Autodesk Inventor part; units mm, degrees
ref_plane "YZ Plane" through (0, 0, 0) normal (1, 0, 0) x (0, 1, 0)
ref_plane "XZ Plane" through (0, 0, 0) normal (0, 1, 0) x (-1, 0, 0)
ref_plane "XY Plane" through (0, 0, 0) normal (0, 0, 1) x (1, 0, 0)
sketch "Sketch1" plane through (0, 0, 0) normal (0, 1, 0) x (-1, 0, 0)
  line L0 (-63.881, 88.9) -> (63.881, 88.9)
  line L1 (63.881, 88.9) -> (63.881, -88.9)
  line L2 (63.881, -88.9) -> (-63.881, -88.9)
  line L3 (-63.881, -88.9) -> (-63.881, 88.9)
  line L4 (-63.881, 88.9) -> (63.881, -88.9) construction
  line L5 (63.881, 88.9) -> (-63.881, -88.9) construction
  point P0 (0, 0)
  dimension "d0" = 127.762
  dimension "d1" = 177.8
extrude "Extrusion1" add sketch "Sketch1" along normal blind 6.35
sketch "Sketch4" plane through (0, 0, 0) normal (0, -1, 0) x (1, 0, 0)
  line L0 (63.881, 88.9) -> (-63.881, 88.9)
  line L1 (-63.881, 88.9) -> (-63.881, -88.9)
  line L2 (63.881, 88.9) -> (-63.881, 88.9)
  line L3 (-63.881, 88.9) -> (-63.881, 76.2)
  line L4 (-63.881, 76.2) -> (63.881, 76.2)
  line L5 (63.881, 76.2) -> (63.881, 88.9)
  point P0 (0, 0)
  point P1 (-59.9113, 88.9)
  point P2 (-63.881, 84.7576)
  dimension "d9" = 12.7
extrude "Extrusion4" cut sketch "Sketch4" against normal blind 6.35
sketch "Sketch6" plane through (0, 0, 0) normal (0, -1, 0) x (1, 0, 0)
  circle A0 centre (-11.3792, 59.9948) radius 1.3716
  circle A1 centre (20.701, 61.722) radius 1.1303
  circle A2 centre (-11.303, 7.62) radius 1.1303
  circle A3 centre (60.071, 7.62) radius 1.1303
  circle A4 centre (-51.181, -41.91) radius 1.4986
  circle A5 centre (50.419, -41.91) radius 1.4986
  circle A6 centre (50.419, -68.58) radius 1.4986
  circle A7 centre (-51.181, -68.58) radius 1.4986
  point P0 (0, 0)
  point P1 (63.881, 76.2)
  dimension "d24" = 2.7432
  dimension "d26" = 2.2606
  dimension "d33" = 2.2606
  dimension "d34" = 2.2606
  dimension "d48" = 2.9972
  dimension "d49" = 2.9972
  dimension "d63" = 2.9972
  dimension "d64" = 2.9972
sketch "Sketch7" plane through (0, 6.35, 0) normal (0, 1, 0) x (1, 0, 0)
  line L0 (-63.881, -76.2) -> (63.881, -76.2)
  line L1 (-63.881, -76.2) -> (-63.881, 88.9)
  line L2 (63.881, -76.2) -> (-63.881, -76.2)
  line L3 (-63.881, -76.2) -> (-63.881, -69.85)
  line L4 (-63.881, -69.85) -> (63.881, -69.85)
  line L5 (63.881, -69.85) -> (63.881, -76.2)
  point P0 (0, 0)
  dimension "d204" = 6.35
extrude "Extrusion7" cut sketch "Sketch7" against normal blind 25.4
sketch "Sketch8" plane through (0, 0, 0) normal (0, -1, 0) x (1, 0, 0)
  circle A0 centre (-20.701, -67.31) radius 1.4986
  circle A1 centre (-20.701, -50.9524) radius 1.4986
  circle A2 centre (16.891, -50.9524) radius 1.4986
  circle A3 centre (16.891, -67.31) radius 1.4986
  point P0 (0, 0)
  point P1 (-63.881, -88.9)
  dimension "d213" = 2.9972
  dimension "d216" = 2.9972
  dimension "d217" = 2.9972
  dimension "d218" = 2.9972
extrude "Extrusion8" cut sketch "Sketch8" against normal blind 25.4
sketch "Sketch9" plane through (0, 6.35, 0) normal (0, 1, 0) x (1, 0, 0)
  point P0 (0, 0)
sketch "Sketch10" plane through (0, 6.35, 0) normal (0, 1, 0) x (1, 0, 0)
  circle A0 centre (-20.701, 67.31) radius 1.4986
  circle A1 centre (-20.701, 67.31) radius 6.35
  circle A2 centre (16.891, 67.31) radius 1.4986
  circle A3 centre (16.891, 67.31) radius 6.35
  circle A4 centre (16.891, 50.9524) radius 1.4986
  circle A5 centre (16.891, 50.9524) radius 6.35
  circle A6 centre (-20.701, 50.9524) radius 1.4986
  circle A7 centre (-20.701, 50.9524) radius 6.35
  point P0 (0, 0)
  dimension "d221" = 12.7
  dimension "d222" = 12.7
  dimension "d223" = 12.7
  dimension "d224" = 12.7
extrude "Extrusion9" cut sketch "Sketch10" against normal blind 3.175
extrude "Extrusion14" cut sketch "Sketch6" against normal blind 6.35 contours A4 | A5 | A6 | A7
sketch "Sketch13" plane through (0, 0, 0) normal (0, -1, 0) x (1, 0, 0)
  circle A0 centre (-51.181, -41.91) radius 1.4986
  circle A1 centre (-51.181, -41.91) radius 6.35
  circle A2 centre (-51.181, -68.58) radius 1.4986
  circle A3 centre (-51.181, -68.58) radius 6.35
  circle A4 centre (50.419, -68.58) radius 1.4986
  circle A5 centre (50.419, -68.58) radius 6.35
  circle A6 centre (50.419, -41.91) radius 1.4986
  circle A7 centre (50.419, -41.91) radius 6.35
  point P0 (0, 0)
  dimension "d247" = 12.7
  dimension "d248" = 12.7
  dimension "d249" = 12.7
  dimension "d250" = 12.7
extrude "Extrusion15" cut sketch "Sketch13" against normal blind 3.175
sketch "Sketch14" plane through (0, 0, 0) normal (0, -1, 0) x (1, 0, 0)
  line L0 (-63.881, -88.9) -> (-63.881, 69.85)
  line L1 (-63.881, 69.85) -> (-38.481, 69.85)
  line L2 (-38.481, 69.85) -> (-38.481, -19.05)
  line L3 (-38.481, -19.05) -> (-63.881, -19.05)
  line L4 (-63.881, -19.05) -> (-63.881, 69.85)
  point P0 (0, 0)
  dimension "d253" = 25.4
  dimension "d254" = 88.9
extrude "Extrusion16" cut sketch "Sketch14" against normal blind 6.35
sketch "Sketch15" plane through (0, 0, 0) normal (0, -1, 0) x (1, 0, 0)
  circle A0 centre (-11.3792, 59.9948) radius 1.3716
  circle A1 centre (40.259, 59.9948) radius 1.3716
  circle A2 centre (-17.7292, 59.9948) radius 1.3716
  circle A3 centre (-17.7292, 10.9982) radius 1.3716
  circle A4 centre (40.259, 10.9982) radius 1.3716
  point P0 (0, 0)
  dimension "d262" = 2.7432
  dimension "d263" = 2.7432
  dimension "d264" = 2.7432
  dimension "d265" = 2.7432
extrude "Extrusion18" cut sketch "Sketch15" against normal blind 25.4 contours A1 | A2 | A3 | A4
hole "Hole17" at (20.701, 0, 61.722) at (60.071, 0, 7.62) at (-11.303, 0, 7.62) direction (0, 1, 0) diameter 2.7432 depth 6.35 countersink diameter 4.1148 countersink angle 82
properties part number "DPLX_P014_Lab_Baseplate_Small_PV" material "Aluminum 6061"
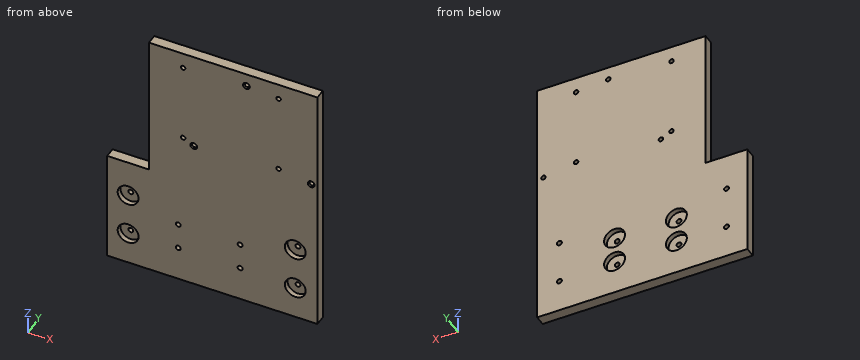
Model file for the job. Use its own axes, mm. Give positions to 0.01 mm unless a question says otherwise; leave off trailing zeros. Loops run counter-clockwise (first coordinate to the right, second up) from the corner with the lowest first, then second, coordinate; pieces in that order, holes last. Notation, with made-up numbers: (-10.5, 57) -> (4.5, 57) arc R32 cw to (4.5, 94) -> close; hole circle Ø8 at (-19, 65). An arc over 180 degrees is marked (long way). Use a Markdown table: item, result. Add a question column.
(1) Slice it at B-B on z = -13. List the corners of the cut face in (x, y), and give its area (3 significant figures).
(2) Drop flat-ended pins along their axis: pin 1 Ø4 at (x, z) = (-52.5, -40.5) entering from -Y (3 decimals); pin 2 Ø6.5 at (x, z) = (-21.5, -64.5) entering from +Y (3 decimals); pin 3 Ø3 at (x, z) = (20.701, 61.722) entering from -Y. Give the stop position or say it passes through.
(3) Wall check: line 1 along X through (y, z) = (2.85, 7.62); line 2 along Z through (x, y) = (-51, 0.5); line 3 along X through (y, z) = (4.8, -68.58). Give the ranges that are in metal, low to high.
(4) Slice it at A-A on y = 4.25. Give the number of separate pieces and of enclosed holes in the cut face, and give its area (3 significant figures).
Filled sheet:
| question | item | result |
|---|---|---|
| 1 | outline | (-38.48, 0) -> (63.88, 0) -> (63.88, 6.35) -> (-38.48, 6.35) -> close |
| 1 | area | 650 mm2 |
| 2 | pin 1 | y = 3.175 |
| 2 | pin 2 | y = 3.175 |
| 2 | pin 3 | y = 0.64 |
| 3 | line 1 | -38.48 to -12.67, -9.93 to 58.7, 61.44 to 63.88 |
| 3 | line 2 | -88.9 to -74.93, -62.23 to -48.26, -35.56 to -19.05 |
| 3 | line 3 | -63.88 to -52.68, -49.68 to -26.92, -14.48 to 10.67, 23.11 to 48.92, 51.92 to 63.88 |
| 4 | separate pieces | 1 |
| 4 | enclosed holes | 15 |
| 4 | area | 17,400 mm2 |
